```python
from build123d import *

# Parameters (mm, degrees)
ESQUISSE1_R        = 1.7
BOSS_EXTRU_1_DEPTH = 2
BOSS_EXTRU_2_START = -2
BOSS_EXTRU_2_DEPTH = 2
CONG_1_R           = 2.5


with BuildPart() as part:
    # Esquisse1 → Boss.-Extru.1 (new body)
    # profile 1 of 2: a face of its own
    with BuildSketch(Plane.XY):
        with BuildLine():
            Line((-6.298682213, 10.443854679), (-3.202171033, 16.875533229))
            Line((-3.202171033, 16.875533229), (-6.531753493, 16.875533229))
            Line((-6.531753493, 16.875533229), (-9.001723843, 11.745225474))
            ThreePointArc((-9.001723843, 11.745225474), (-10.480816133, 9.976643404), (-12.62301596, 9.124248871))
            Line((-12.62301596, 9.124248871), (-59.336252698, 2.974334584))
            ThreePointArc((-59.336252698, 2.974334584), (-61.944674121, 0), (-59.336252698, -2.974334584))
            Line((-59.336252698, -2.974334584), (-1.395824109, -10.602336719))
            ThreePointArc((-1.395824109, -10.602336719), (5.08555675, -9.407177121), (9.635283697, -4.638876688))
            Line((9.635283697, -4.638876688), (19.993327919, 16.875533229))
            Line((19.993327919, 16.875533229), (16.663745459, 16.875533229))
            Line((16.663745459, 16.875533229), (6.932242067, -3.337505893))
            ThreePointArc((6.932242067, -3.337505893), (3.658876225, -6.768127543), (-1.004245533, -7.628002135))
            Line((-1.004245533, -7.628002135), (-51.413902738, -0.991444861))
            ThreePointArc((-51.413902738, -0.991444861), (-52.283376546, 0), (-51.413902738, 0.991444861))
            Line((-51.413902738, 0.991444861), (-12.231437384, 6.149914287))
            ThreePointArc((-12.231437384, 6.149914287), (-8.721875965, 7.546390437), (-6.298682213, 10.443854679))
        make_face()
    # profile 2 of 2: a face of its own
    with BuildSketch(Plane.XY):
        with BuildLine():
            Line((16.663745459, 16.875533229), (-3.202171033, 16.875533229))
            Line((-3.202171033, 16.875533229), (-6.298682213, 10.443854679))
            ThreePointArc((-6.298682213, 10.443854679), (-8.721875965, 7.546390437), (-12.231437384, 6.149914287))
            Line((-12.231437384, 6.149914287), (-51.413902738, 0.991444861))
            ThreePointArc((-51.413902738, 0.991444861), (-52.283376546, 0), (-51.413902738, -0.991444861))
            Line((-51.413902738, -0.991444861), (-1.004245533, -7.628002135))
            ThreePointArc((-1.004245533, -7.628002135), (3.658876225, -6.768127543), (6.932242067, -3.337505893))
            Line((6.932242067, -3.337505893), (16.663745459, 16.875533229))
        make_face()
        with Locations((0.467987162, 12.175533229)):
            Circle(ESQUISSE1_R, mode=Mode.SUBTRACT)
        with Locations((8.467987162, 12.175533229)):
            Circle(ESQUISSE1_R, mode=Mode.SUBTRACT)
    extrude(amount=BOSS_EXTRU_1_DEPTH)

    # Esquisse1<5> → Boss.-Extru.2 (add)
    with BuildSketch(Plane.XY.offset(BOSS_EXTRU_2_START)):
        with BuildLine():
            Line((-6.298682213, 10.443854679), (-3.202171033, 16.875533229))
            Line((-3.202171033, 16.875533229), (-6.531753493, 16.875533229))
            Line((-6.531753493, 16.875533229), (-9.001723843, 11.745225474))
            ThreePointArc((-9.001723843, 11.745225474), (-10.480816133, 9.976643404), (-12.62301596, 9.124248871))
            Line((-12.62301596, 9.124248871), (-59.336252698, 2.974334584))
            ThreePointArc((-59.336252698, 2.974334584), (-61.944674121, 0), (-59.336252698, -2.974334584))
            Line((-59.336252698, -2.974334584), (-1.395824109, -10.602336719))
            ThreePointArc((-1.395824109, -10.602336719), (5.08555675, -9.407177121), (9.635283697, -4.638876688))
            Line((9.635283697, -4.638876688), (19.993327919, 16.875533229))
            Line((19.993327919, 16.875533229), (16.663745459, 16.875533229))
            Line((16.663745459, 16.875533229), (6.932242067, -3.337505893))
            ThreePointArc((6.932242067, -3.337505893), (3.658876225, -6.768127543), (-1.004245533, -7.628002135))
            Line((-1.004245533, -7.628002135), (-51.413902738, -0.991444861))
            ThreePointArc((-51.413902738, -0.991444861), (-52.283376546, 0), (-51.413902738, 0.991444861))
            Line((-51.413902738, 0.991444861), (-12.231437384, 6.149914287))
            ThreePointArc((-12.231437384, 6.149914287), (-8.721875965, 7.546390437), (-6.298682213, 10.443854679))
        make_face()
    extrude(amount=BOSS_EXTRU_2_DEPTH)

    # Congé1
    # the kernel refuses this fillet: 2.5 mm, written as the material it takes off along each edge
    with BuildSketch(Plane(origin=(22.913745459, 16.875533229, 0), x_dir=(0, 0, 1), z_dir=(-1, 0, 0))) as cong_1_piece_1_section:
        with BuildLine():
            CenterArc((CONG_1_R, -CONG_1_R), CONG_1_R, 90, 90)
            Line((0, -CONG_1_R), (0, 0))
            Line((0, 0), (CONG_1_R, 0))
        make_face()
    cong_1_piece_1 = extrude(amount=32.365916492, mode=Mode.PRIVATE)
    cong_1_piece_1 = split(cong_1_piece_1, bisect_by=Plane(origin=(14.522128014, 12.4272383, 0.565987786), z_dir=(-0.9010138766913354, 0.4337902650010155, 0)), keep=Keep.TOP, mode=Mode.PRIVATE)
    cong_1_piece_1 = split(cong_1_piece_1, bisect_by=Plane(origin=(-1.605539627, 20.191852587, 0.565987786), z_dir=(0.9010138766913354, -0.4337902650010154, 0)), keep=Keep.TOP, mode=Mode.PRIVATE)
    add(cong_1_piece_1, mode=Mode.SUBTRACT)


solid = part.part
```
CAD build for the part. Positions are in the model's coordinates, mm. A direction names the side the tool comes from. Coordinates: 2 decimals unless noted, no trailing zeros. Order: outer loops, then holes, each group sorted by start corner. A loop starts at its lowest first (then second) coordinate and runs counter-clockwise, first axis right, second up.
(1) Mould opens along Y. For faces 4 (the face through (-61.944, 0.06, -0.028)), 5 (the face through (-12, 3, 2)), 6 (the face through (18, 16.876, 0)), 7 (the face through (-32.097, 3.535, -1.014)) say: released by +Y, released by -Y, zero draft, split by the parting line, or undercut.
Solution:
face 4: split by the parting line
face 5: zero draft
face 6: released by +Y
face 7: undercut
(2) Saw through at B-B, the plane y = 1.75. Write the cut outline in (x, z).
Solution:
outline: (-61.38, -2) - (-45.65, -2) - (-45.65, 0) - (9.38, 0) - (9.38, -2) - (12.71, -2) - (12.71, 2) - (-61.38, 2) - close
(3) Pin check, flat tips, straight feed: pin 1 Ø4.5 at (x, y) = (8.47, 12.18) entering from +Z; pin 2 Ø5.5 at (x, y) = (0.47, 12.18) entering from -Z. Stop position of each tip, or through.
Solution:
pin 1: stops at z = 2
pin 2: stops at z = 0
(4) Saw through at A-A, the plane z = 0.95. Write the cut outline in (x, y).
Solution:
outline: (-59.34, -2.97) - (-1.4, -10.6) arc R10.69 ccw to (9.64, -4.64) - (19.99, 16.88) - (16.66, 16.88) - (16.4, 16.34) - (-3.46, 16.34) - (-3.2, 16.88) - (-6.53, 16.88) - (-9, 11.75) arc R4.7 cw to (-12.62, 9.12) - (-59.34, 2.97) arc R3 ccw to start; hole circle Ø3.4 at (0.47, 12.18); hole circle Ø3.4 at (8.47, 12.18)
(5) Saw through at C-C, the plane x = -35. Write the cut outline in (y, z).
Solution:
outline: (-6.18, -2) - (-3.15, -2) - (-3.15, 0) - (3.15, 0) - (3.15, -2) - (6.18, -2) - (6.18, 2) - (-6.18, 2) - close
(6) Which spindle directions (+Z, -Z, +X, -X, +Y, -Y) get a long thin tool onto all of the face, cutting with end or side? Do faces 1 (the face through (-11, 3, 0)), 2 (the face through (-7.749, 14.346, -0.028)), 3 (the face through (3.718, -6.736, -1.014)). Say none if no direction does.
Solution:
face 1: -Z
face 2: +Z, -Z, -X, +Y
face 3: -Z, +Y
(7) Drill centre lines: L1, parallel to Y at x = -11.5, z = -0.45; L2, parallel to Z at x = -5.5, y = 6; L3, parallel to Y at x = -3.5, z = -0.55. Where is each one in solid material? Low to high.
Solution:
L1: y = -9.27 to -6.25, 6.28 to 9.42
L2: z = 0 to 2
L3: y = -10.33 to -7.3, 16.26 to 16.88
